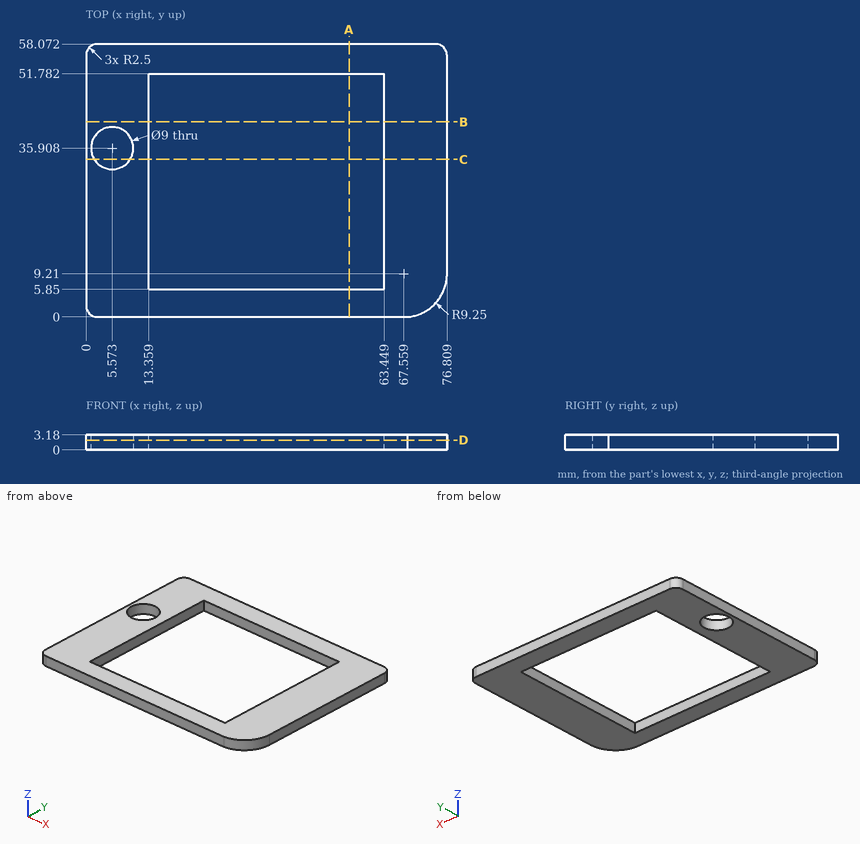
Print and shaded views of the part. All mm, measured from the part's lowest x, y and z. Coordinates: 2 decimals unless noted, no trailing zeros. Order: outer loops, then holes, each group sorted by start corner. A loop starts at its lowest first (then second) coordinate and runs counter-clockwise, first axis right, second up. Notation, with made-up numbers: M 87.5,76.5 L 100.5,76.5 A16 ccw 100.5,87.5 Z; hole C -10.5,86 d5. An arc over 180 degrees is marked long. One line per question, with ' | ' between items. Start each with the question number.
Q1. Flat gauge pin, fed straight in: pin 1 Ø5 at (x, y) = (46.5, 49) entering from +Z. Where does the tip first touch, or does it go through?
Q2. Saw through at C-C (y = 33.5). Count the separate pieces of the cut face and the enclosed holes in it.
Q3. Saw through at B-B (y = 41.5). List the corners of the cut face in (x, z).
Q4. Saw through at A-A (x = 56). List the corners of the cut face in (y, z).
Q5. Saw through at D-D (z = 2.1). List the corners of the cut face in (x, y), then the cut area to 3 significant figures.
Q6. Probe L1, parallel to X at y = 41.5, z = 1.3; L2, parallel to Y at x = 44, z = 0.8. List the from-to ranges inside material, lowest first. Write a range as from..to.
Check values:
1) pin 1: passes through
2) separate pieces: 3 | enclosed holes: 0
3) outline: M 0,0 L 13.36,0 L 13.36,3.18 L 0,3.18 Z; M 63.45,0 L 76.81,0 L 76.81,3.18 L 63.45,3.18 Z
4) outline: M 0,0 L 5.85,0 L 5.85,3.18 L 0,3.18 Z; M 51.78,0 L 58.07,0 L 58.07,3.18 L 51.78,3.18 Z
5) outline: M 0,2.5 A2.5 ccw 2.5,0 L 68.42,0 A9.25 ccw 76.81,9.25 L 76.81,55.57 A2.5 ccw 74.31,58.07 L 2.5,58.07 A2.5 ccw 0,55.57 Z; hole C 5.57,35.91 d9; hole M 13.36,5.85 L 63.45,5.85 L 63.45,51.78 L 13.36,51.78 Z | area: 2,070 mm2
6) L1: x = 0..13.36, 63.45..76.81 | L2: y = 0..5.85, 51.78..58.07
